from build123d import *

# Parameters (mm, degrees)
SKETCH1_R           = 25
BOSS_EXTRUDE1_DEPTH = 100
SKETCH2_R           = 80
BOSS_EXTRUDE2_DEPTH = 70
DRAFT1_ANGLE        = 35
SKETCH4_W           = 50
SKETCH4_H           = 50
CUT_EXTRUDE1_DEPTH  = 50


with BuildPart() as part:
    # Sketch1 → Boss-Extrude1 (new body)
    with BuildSketch(Plane(origin=(0, 0, 0), x_dir=(1, 0, 0), z_dir=(0, 1, 0))):
        with Locations(Location((0, 0, 0), (0, 0, 90))):
            Circle(SKETCH1_R)
    extrude(amount=BOSS_EXTRUDE1_DEPTH)

    # Sketch2 → Boss-Extrude2 (add)
    with BuildSketch(Plane(origin=(0, 0, 0), x_dir=(1, 0, 0), z_dir=(0, 1, 0))):
        with Locations(Location((0, 0, 0), (0, 0, 270))):
            Circle(SKETCH2_R)
    extrude(amount=BOSS_EXTRUDE2_DEPTH)

    # Draft1
    draft1_faces = [part.faces().sort_by_distance(p)[0] for p in [
        (0, 35, -80),
    ]]
    draft(draft1_faces, Plane.ZX.offset(70), DRAFT1_ANGLE)

    # Sketch4 → Cut-Extrude1 (cut)
    with BuildSketch(Plane.XZ):
        Rectangle(SKETCH4_W, SKETCH4_H)
    extrude(amount=-CUT_EXTRUDE1_DEPTH, mode=Mode.SUBTRACT)


solid = part.part
Geometry: final body of the model. Coordinates: model frame, mm. A direction names the side the tool comes from. Coordinates: 2 decimals unless noted, no trailing zeros. Loops run counter-clockwise (first coordinate to the right, second up) from the corner with the lowest first, then second, coordinate; pieces in that order, holes last. Notation, with made-up numbers: M 82.25,6 L 118.25,6 A18 cw 118.25,14 Z; hole C 5.5,-9.5 d6. An arc over 180 degrees is marked long. One line per item, written item: value. Start each with the question number.
1) Material intervals for L1, parallel to Z at x = 21, y = 21; L2, parallel to Z at x = -1, y = 75; L3, parallel to X at y = 32, z = -13.5, sorted ascending. Write a range as from..to.
2) Cut plane D-D (y = 45). Return loops of the section in (x, z), then the cut area to 3 significant figures.
3) Pin query (flat end, axial travel): P1, Ø4, axis at x = 53, z = -51, coming from the +Y side; P2, Ø3, axis at x = 82.5, y = 36, coming from the +Z side; P3, Ø12, axis at x = 67, y = 13, coming from the +Z side; P4, Ø6, axis at x = -77, z = -45, coming from the -Y side. Return the tip coordinate at first contact, or that it passes through.
4) Cut plane A-A (z = 0). Return loops of the section in (x, y).
5) Cut plane B-B (x = 0). Return loops of the section in (y, z).
6) Reachability of faces 1 (the flat face through (25, 25, 0)), 2 (the flat face through (19, 70, 17)), 3 (the flat face through (-27, 0, -2)) from +Z, -Z, +X, -X, +Y, -Y: full face, straight path, thin tool, end or side. Return the list, or none.
7) Draft query along X for faces 4 (the flat face through (0, 25, 25)), 5 (the flat face through (0, 100, 0)), 6 (the conical face through (-81.09, 65.62, -18.01)). Return one class per face: released by +X, released by -X, zero draft, split by the parting line, or undercut.
8) Cut plane C-C (y = 13). Return loops of the section in (x, z), then the cut area to 3 significant figures.
Evaluation:
1. L1: -112.36..-25, 25..112.36
1. L2: -24.98..24.98
1. L3: -105.75..-25, 25..105.75
2. outline: C 0,0 d195.01; hole M -25,-25 L 25,-25 L 25,25 L -25,25 Z
2. area: 27,400 mm^2
3. P1: y = 70
3. P2: z = 65.56
3. P3: z = 105.72
3. P4: y = 0
4. outline: M -129.01,0 L -25,0 L -25,50 L 25,50 L 25,0 L 129.01,0 L 80,70 L 25,70 L 25,100 L -25,100 L -25,70 L -80,70 Z
5. outline: M 0,-129.01 L 70,-80 L 70,-25 L 100,-25 L 100,25 L 70,25 L 70,80 L 0,129.01 L 0,25 L 50,25 L 50,-25 L 0,-25 Z
6. face 1: -Y
6. face 2: +Y
6. face 3: +Z, -Z, +X, -X, -Y
7. face 4: undercut
7. face 5: zero draft
7. face 6: split by the parting line
8. outline: C 0,0 d239.82; hole M -25,-25 L 25,-25 L 25,25 L -25,25 Z
8. area: 42,700 mm^2
